Check sheet for the drawn part. Datum: minimum x, y, z corner. Units: mm. Coordinates: 2 decimals unless noted, no trailing zeros. Loops run counter-clockwise (first coordinate to the right, second up) from the corner with the lowest first, then second, coordinate; pieces in that order, holes last.
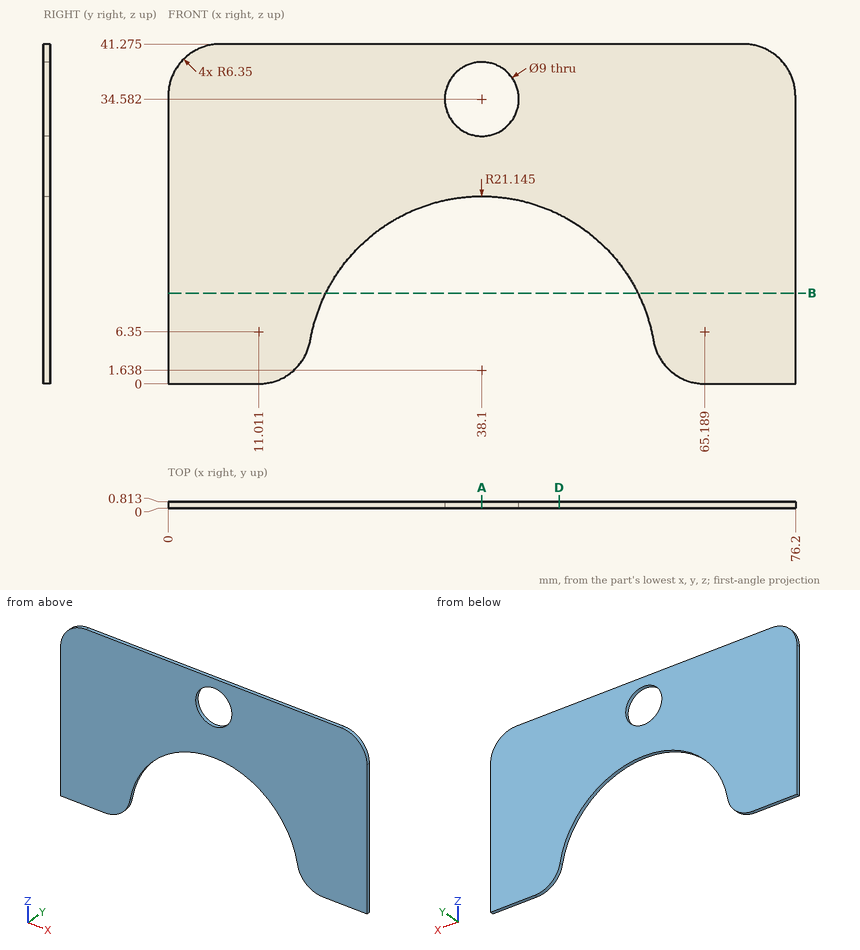
1) Section check D-D on x = 47.5. Enter the section's corners in (y, z) (1 decimal).
Answer sheet:
outline: (0, 20.6) - (0.8, 20.6) - (0.8, 41.3) - (0, 41.3) - close
2) Section check B-B on z = 11. Enter the section's corners in (x, y).
Answer sheet:
outline: (0, 0) - (19.14, 0) - (19.14, 0.81) - (0, 0.81) - close; (57.06, 0) - (76.2, 0) - (76.2, 0.81) - (57.06, 0.81) - close
3) Section check A-A on x = 38.1. Enter the section's corners in (y, z) (1 decimal).
Answer sheet:
outline: (0, 22.8) - (0.8, 22.8) - (0.8, 30.1) - (0, 30.1) - close; (0, 39.1) - (0.8, 39.1) - (0.8, 41.3) - (0, 41.3) - close
4) Scan lines: line 1 (Z direction, x = 38.1, y = 0.2) (1 decimal); line 2 (X direction, y = 0.65, z = 18) (1 decimal); line 3 (Z direction, x = 35.5, y = 0.5) (1 decimal). Record each from-to range of solid material in increasing order.
Answer sheet:
line 1: z = 22.8 to 30.1, 39.1 to 41.3
line 2: x = 0 to 24.7, 51.5 to 76.2
line 3: z = 22.6 to 30.9, 38.3 to 41.3
5) Depth check by flat-ended pin: pin 1 (10.5 mm diameter, centred on x = 38.1, z = 34.58, fed in from -Y); pin 2 (3 mm diameter, centred on x = 56, z = 7.5, fed in from -Y). Enter the tip coordinate at first touch or a pass-through.
Answer sheet:
pin 1: stops at y = 0
pin 2: passes through
